```python
from build123d import *

# Parameters (mm, degrees)
PAD_DEPTH            = 25
SKETCH002_R          = 2
SKETCH003_R          = 1.300458
POCKET_DEPTH         = 2
SKETCH004_R          = 1.5
POCKET001_DEPTH      = 8
SKETCH005_R          = 1.5000493445
POCKET002_DEPTH      = 6.5
POCKET002_DEPTH_BACK = 6.5


with BuildPart() as part:
    # Sketch → Pad (new body)
    with BuildSketch(Plane.XY):
        Polygon((-0.5039697873, 14.7133968199), (-12.9849027673, 7.508821487), (-12.99, -7.5), (0, -14.9996699964), (12.99, -7.5), (12.99, 7.5), (12.74, 7.0669872981), align=None)
        Polygon((0, 13.4996699964), (-11.6910571596, 6.7498349982), (-11.6910571596, -6.7498349982), (0, -13.4996699964), (11.6910571596, -6.7498349982), (11.6910571596, 6.7498349982), align=None, mode=Mode.SUBTRACT)
    extrude(amount=PAD_DEPTH)

    # Sketch001 (on Face14 of Pad) → AdditiveLoft section 0
    with BuildSketch(Plane(origin=(0, 0, 0), x_dir=(1, 0, 0), z_dir=(0, 0, -1))):
        Polygon((0, 15.7996699964), (-13.6829155883, 7.8998349982), (-13.6829155883, -7.8998349982), (0, -15.7996699964), (13.6829155883, -7.8998349982), (13.6829155883, 7.8998349982), align=None)
    # Sketch002 → AdditiveLoft section 1
    with BuildSketch(Plane.XY.offset(-66)):
        Circle(SKETCH002_R)
    loft()

    # Sketch003 (on Face24 of AdditiveLoft) → Pocket (cut)
    with BuildSketch(Plane.XY):
        with Locations((4.766006, 8.46789)):
            Circle(SKETCH003_R)
    extrude(amount=-POCKET_DEPTH, mode=Mode.SUBTRACT)

    # Sketch004 (on Face24 of Pocket) → Pocket001 (cut)
    with BuildSketch(Plane.XY):
        with Locations((0, 5)):
            Circle(SKETCH004_R)
        with Locations((0, -5)):
            Circle(SKETCH004_R)
    extrude(amount=-POCKET001_DEPTH, mode=Mode.SUBTRACT)

    # Sketch005 → Pocket002 (cut, two sides)
    with BuildSketch(Plane.XZ) as pocket002_sk:
        with Locations((0, -8.012167)):
            Circle(SKETCH005_R)
    extrude(amount=-POCKET002_DEPTH, mode=Mode.SUBTRACT)
    extrude(pocket002_sk.sketch, amount=POCKET002_DEPTH_BACK, mode=Mode.SUBTRACT)

    # Sketch006 → Revolution (revolve)
    with BuildSketch(Plane.XZ):
        with BuildLine():
            Line((0, -66), (2, -66))
            ThreePointArc((0, -68), (1.4142135624, -67.4142135624), (2, -66))
            Line((0, -66), (0, -68))
        make_face()
    revolve(axis=Axis((0, 0, 0), (0, 0, 1)))


solid = part.part
```
The model under review builds one solid part; all positions refer to its coordinate system, in mm. A direction names the side the tool comes from. Coordinates: 2 decimals unless noted, no trailing zeros. One line per question, with ' | ' between items.
(1) For probe 1 along Y at (x, z) = (0, -5); probe 2 along Y at (x, z) = (4, 2.5); probe 3 along X at (y, z) = (9, 5), list the stretches that pass through material, from the lowest coordinate up. Write a range as from..to.
Geometry results:
probe 1: y = -14.75..-6.5, -3.5..3.5, 6.5..14.75 | probe 2: y = -12.69..-11.19, 11.19..12.11 | probe 3: x = -10.4..-7.79, 7.79..9.39
(2) Insertion check: pin 1 (12 mm diameter, centred on x = 7, y = 1, fed in from -Z); pin 2 (5 mm diameter, centred on x = -9.5, z = -3, fed in from -Y); pin 3 (0.9 mm diameter, centred on x = 0, z = -7.5, fed in from -Y). Each pin has a flat end and moves straight along its axis. Give the tip position at first contact, or say it passes through.
Geometry results:
pin 1: stops at z = -67.69 | pin 2: stops at y = -11.23 | pin 3: stops at y = -14.33
(3) The part is to be moulded in two halves that separate along Y. For faces 1 (the face through (0.806, 6.265, -3.95)), 2 (the face through (-5.764, 10.172, 12.325)), 3 (the face through (6.211, 10.837, 12.325)), 4 (the face through (12.99, 0, 12)), say which applies: +Y half, -Y half, draft (parallel to the pull), parting line (faces both ways), or undercut.
Geometry results:
face 1: undercut | face 2: undercut | face 3: +Y half | face 4: draft
(4) Machinability: for faces 5 (the face through (-5.927, -10.078, 12.325)), 6 (the face through (6.404, -11.302, 12.325)), 7 (the face through (-6.586, -11.197, 12.325)), which of the approach directions +Z, -Z, +X, -X, +Y, -Y give a long, thin tool a straight path to every point of the face, cutting with its end or side? Answer none if there is none.
Geometry results:
face 5: +Z | face 6: +Z, +X, -Y | face 7: +Z, -X, -Y
